Here's the drawing with two shaded views (mm, measured from the low corner). I have some questions. A direction names the side the tool comes from. Round coordinates to 2 decimals unless told otherwise and drop trailing zeros. Write each loop counter-clockwise with the first axis right and the second up, starting at its lowest first coordinate (ties: lowest second). Pieces come first, ordered by that corner, then holes. Notation, with made-up numbers: M 27.5,-10.5 L 54.5,-10.5 A18 cw 54.5,22.5 Z; hole C 42,53 d6. An arc over 180 degrees is marked long. Write item = value, one per line. Start each with the question number.
(1) On a 3-axis mill with a long thin cutter (end or side, diameter ignored), from which of +Z, -Z, +X, -X, +Y, -Y can I reach the whole of each face in a straight line? I mean the marked faces 5, 6 and 7. Say none if no direction works.
(2) I want a section at B-B (y = 14.25). List the corners of the cut face in (x, z) for me.
(3) I want a section at A-A (z = 10.25). List the corners of the cut face in (x, y) for me.
(4) I want a section at D-D (z = 8.5). List the corners of the cut face in (x, y) for me.
(5) If we mould it in two halves opening along Y, with no side actions, what happens to the marked faces 1, 2, 3 and 4? For each: released by +Y, released by -Y, zero draft, split by the parting line, or undercut.
(6) Will this pin go through, and if not, where does the flat tip stop? pin 1 Ø4.5 at (x, y) = (7.78, 7.88) entering from -Z.
(7) I need wall thicknesses on line 1 along X through (y, z) = (3.5, 1); line 2 along Y through (x, z) = (7.5, 4.5) (1 decimal). Which ranges of each line are inside material? Lowest first, please.
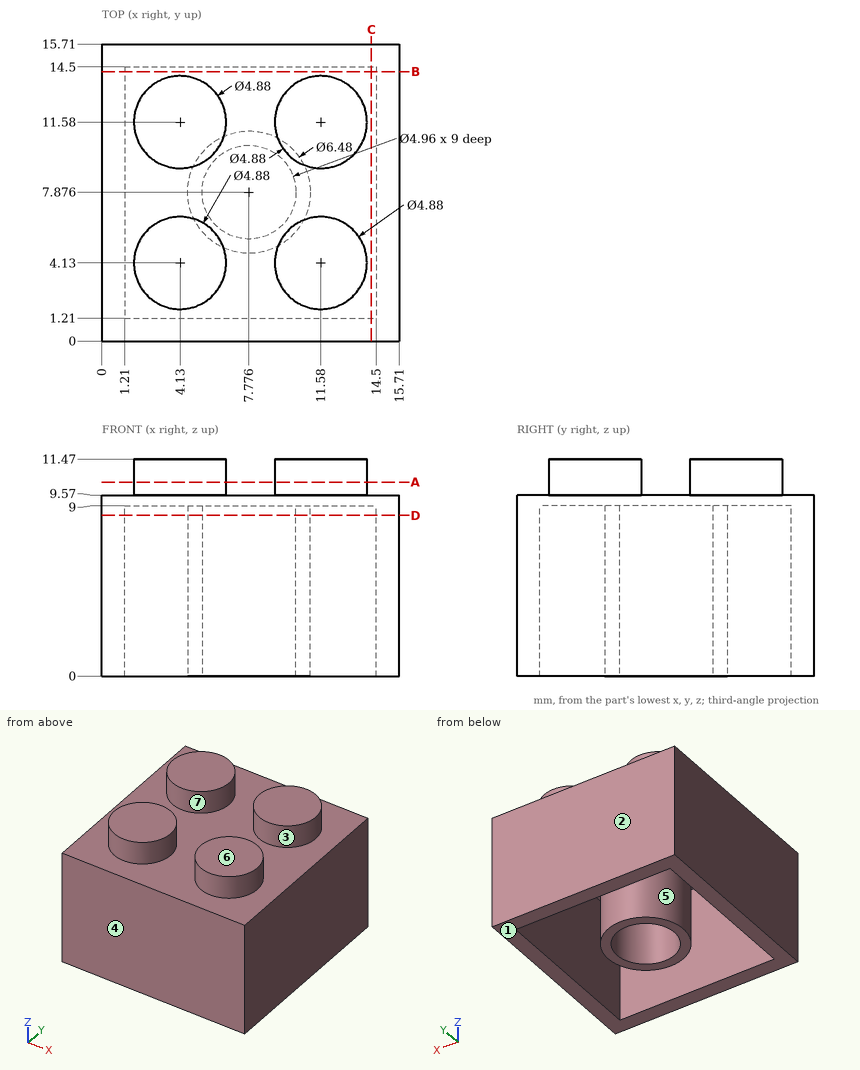
Returned:
q1.face_5 = -Z
q1.face_6 = +Z, +X, -X, +Y, -Y
q1.face_7 = +Z
q2.outline = M 0,0 L 1.21,0 L 1.21,9 L 14.5,9 L 14.5,0 L 15.71,0 L 15.71,9.57 L 0,9.57 Z
q3.outline = C 4.13,4.13 d4.88; C 4.13,11.58 d4.88; C 11.58,4.13 d4.88; C 11.58,11.58 d4.88
q4.outline = M 0,0 L 15.71,0 L 15.71,15.71 L 0,15.71 Z; C 7.78,7.88 d6.48; hole M 1.21,1.21 L 14.5,1.21 L 14.5,14.5 L 1.21,14.5 Z; hole C 7.78,7.88 d4.96
q5.face_1 = zero draft
q5.face_2 = released by +Y
q5.face_3 = undercut
q5.face_4 = released by -Y
q6.pin_1 = 9
q7.line_1 = 0 to 1.21, 14.5 to 15.71
q7.line_2 = 0 to 1.2, 4.6 to 5.4, 10.3 to 11.1, 14.5 to 15.7
